Build history of the part. All positions in model axes, mm. A direction names the side the tool comes from. Give positions to 0.01 mm unless a question says otherwise; leave off trailing zeros. Order: outer loops, then holes, each group sorted by start corner. A loop starts at its lowest first (then second) coordinate and runs counter-clockwise, first axis right, second up. Notation, with made-up numbers: (78.5, -19) - (122.5, -19) arc R36 cw to (122.5, 15) - close; hole circle Ø7 at (-6.75, -35.5). An arc over 180 degrees is marked (long way). Answer in a Markdown table with one row per item.
```python
from build123d import *

# Parameters (mm, degrees)
SKETCH2_W           = 60
SKETCH2_H           = 30
SKETCH2_R           = 6
BOSS_EXTRUDE1_DEPTH = 28
BOSS_EXTRUDE2_DEPTH = 20


with BuildPart() as part:
    # Sketch2 → Boss-Extrude1 (new body)
    with BuildSketch(Plane.XY):
        with Locations((30, 15)):
            Rectangle(SKETCH2_W, SKETCH2_H)
        with Locations((44, 16)):
            Circle(SKETCH2_R, mode=Mode.SUBTRACT)
    extrude(amount=BOSS_EXTRUDE1_DEPTH)

    # Sketch2_3 → Boss-Extrude2 (add)
    with BuildSketch(Plane.XY):
        Polygon((35.673729326, 39.1665834), (35.673729326, 50), (20, 50), (20, 75), (0, 75), (0, 50), (0, 30), (47.673729326, 30), (47.673729326, 39.1665834), align=None)
    extrude(amount=BOSS_EXTRUDE2_DEPTH)


solid = part.part
```
1. Cut at C-C on z = 11.5. Write the cut outline in (x, y).
Check result:
| item | result |
|---|---|
| outline | (0, 0) - (60, 0) - (60, 30) - (47.67, 30) - (47.67, 39.17) - (35.67, 39.17) - (35.67, 50) - (20, 50) - (20, 75) - (0, 75) - close; hole circle Ø12 at (44, 16) |
2. Two-plate mould, pull along Y, no slides. Class faces 4 (the face through (38, 16, 14)), 5 (the face through (30, 0, 14)), 6 (the face through (10, 75, 10)), 7 (the face through (35.674, 45, 10)): +Y half, -Y half, draft (parallel to the pull), parting line (faces both ways), or undercut.
Check result:
| item | result |
|---|---|
| face 4 | undercut |
| face 5 | -Y half |
| face 6 | +Y half |
| face 7 | draft |
3. Which spindle directions (+Z, -Z, +X, -X, +Y, -Y) get a long thin tool onto all of the face, cutting with end or side? Do faces 1 (the face through (23, 30, 0)), 2 (the face through (18, 48, 20)), 3 (the face through (20, 62, 10)). Say none if no direction does.
Check result:
| item | result |
|---|---|
| face 1 | -Z, +X, -X, +Y, -Y |
| face 2 | +Z, +X, -X, +Y |
| face 3 | +Z, -Z, +X, +Y |
4. Cut at B-B on x = 44. Write the cut outline in (y, z).
Check result:
| item | result |
|---|---|
| outline | (0, 0) - (10, 0) - (10, 28) - (0, 28) - close; (22, 0) - (39.17, 0) - (39.17, 20) - (30, 20) - (30, 28) - (22, 28) - close |
5. Probe line 1 (Y direction, x = 44, z = 18.5); line 2 (X direction, y = 37.5, z = 2.25); line 3 (Y direction, x = 45, z = 24.5). List the from-to ranges inside material, lowest first.
Check result:
| item | result |
|---|---|
| line 1 | y = 0 to 10, 22 to 39.17 |
| line 2 | x = 0 to 47.67 |
| line 3 | y = 0 to 10.08, 21.92 to 30 |
6. Drop flat-ended pins along their axis: P1, Ø13.5, axis at x = 20.5, y = 41.5, coming from the +Z side; P2, Ø2.5, axis at y = 33.5, z = 12.5, coming from the +X side; P3, Ø1.5, axis at x = 34.5, z = 20.5, coming from the +Y side; P4, Ø6, axis at y = 31, z = 18.5, coming from the +X side. Give the stop position or say it passes through.
Check result:
| item | result |
|---|---|
| P1 | stops at z = 20 |
| P2 | stops at x = 47.67 |
| P3 | stops at y = 50 |
| P4 | stops at x = 60 |
7. Cut at D-D on x = 27. Write the cut outline in (y, z), and give its area (3 significant figures).
Check result:
| item | result |
|---|---|
| outline | (0, 0) - (50, 0) - (50, 20) - (30, 20) - (30, 28) - (0, 28) - close |
| area | 1,240 mm² |
8. Cut at A-A on y = 16. Write the cut outline in (x, z).
Check result:
| item | result |
|---|---|
| outline | (0, 0) - (38, 0) - (38, 28) - (0, 28) - close; (50, 0) - (60, 0) - (60, 28) - (50, 28) - close |
